from build123d import *

# Parameters (mm, degrees)
F0_W     = 203.2
F0_H     = 203.2
F1_DEPTH = 3.175
F2_W     = 187.96
F2_H     = 187.96
F3_DEPTH = 3.175
F4_R     = 17.4625
F5_DEPTH = 25.4


with BuildPart() as f1:
    # F0 (on Top) → F1 (new body)
    with BuildSketch(Plane.XY):
        Rectangle(F0_W, F0_H)
    extrude(amount=F1_DEPTH)

    # F2 (on face) → F3 (join)
    with BuildSketch(Plane.XY.offset(3.175)):
        Rectangle(F2_W, F2_H)
    extrude(amount=F3_DEPTH)

    # F4 (on face) → F5 (cut)
    with BuildSketch(Plane.XY.offset(6.35)):
        Circle(F4_R)
    extrude(amount=-F5_DEPTH, mode=Mode.SUBTRACT)


solid = f1.part
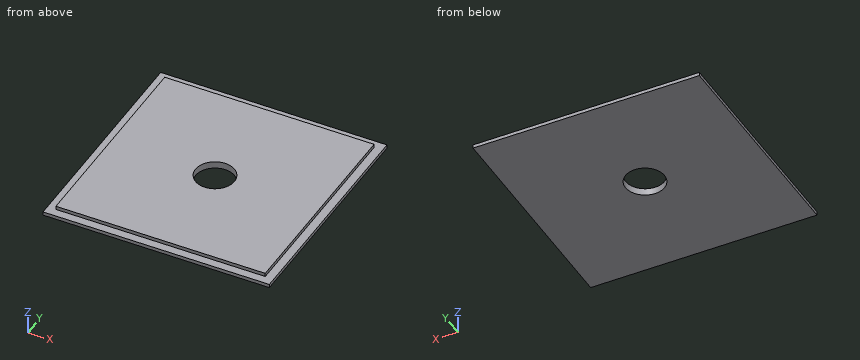
Work out the finished part from the listing and answer in its coordinate system (mm). Give positions to 0.01 mm unless a question says otherwise; leave off trailing zeros. Loops run counter-clockwise (first coordinate to the right, second up) from the corner with the lowest first, then second, coordinate; pieces in that order, holes last. Notation, with made-up numbers: (71.5, -27) -> (101.5, -27) arc R28 cw to (101.5, 11) -> close; hole circle Ø7 at (17, 19.25). An arc over 180 degrees is marked (long way). Use a Markdown table: item, result. Add a question column.
1. Flat-ended cylindrical pins translate along their axes: pin 1 Ø1 at (y, z) = (40.5, 5) entering from +X; pin 2 Ø1 at (y, z) = (-29, 4.5) entering from -X; pin 3 Ø1.6 at (x, z) = (-24, 5.5) entering from +Y. Find the tip coordinate at first contact, or state that the pin passes through.
2. Section C-C on z = 5 is taken. Determine the outline of the cut face in (x, y) (1 decimal).
3. Section D-D on x = -37 is taken. Determine the outline of the cut face in (y, z) (3 decimals).
4. Find the intervals of material crossed by probe 1 along Y at (x, z) = (0, 4.75); probe 2 along Y at (x, z) = (1, 3); probe 3 along X at (y, z) = (75.5, 5), in increasing order.
Results below:
| question | item | result |
|---|---|---|
| 1 | pin 1 | stops at x = 93.98 |
| 1 | pin 2 | stops at x = -93.98 |
| 1 | pin 3 | stops at y = 93.98 |
| 2 | outline | (-94, -94) -> (94, -94) -> (94, 94) -> (-94, 94) -> close; hole circle Ø34.9 at (0, 0) |
| 3 | outline | (-101.6, 0) -> (101.6, 0) -> (101.6, 3.175) -> (93.98, 3.175) -> (93.98, 6.35) -> (-93.98, 6.35) -> (-93.98, 3.175) -> (-101.6, 3.175) -> close |
| 4 | probe 1 | y = -93.98 to -17.46, 17.46 to 93.98 |
| 4 | probe 2 | y = -101.6 to -17.43, 17.43 to 101.6 |
| 4 | probe 3 | x = -93.98 to 93.98 |
